Geometry: final body of the model. Coordinates: model frame, mm. Round coordinates to 2 decimals unless told otherwise and drop trailing zeros. Order: outer loops, then holes, each group sorted by start corner. A loop starts at its lowest first (then second) coordinate and runs counter-clockwise, first axis right, second up. Notation, with made-up numbers: (43.5, 67.5) - (66.5, 67.5) arc R18 cw to (66.5, 92.5) - close; hole circle Ø10 at (12.25, 54). An arc over 180 degrees is marked (long way). Put each result on its own line as item: value. Start each with the question number.
(1) Section A-A (z = 25). Output: boundary loops of the cut face in (x, y).
(2) Section B-B (x = -14). Output: boundary loops of the cut face in (y, z).
(3) Pin query (flat end, axial travel): P1, Ø2, axis at x = 46.5, y = 4, coming from the -Z side; P2, Ø2.5, axis at y = 5, z = -2.5, coming from the +X side; P3, Ø1, axis at y = 6, z = -6, coming from the -X side. Return the tip coordinate at first contact, or that it passes through.
(4) Material intervals for L1, parallel to Z at x = 15, y = 4.75; L2, parallel to X at y = 2.75, z = 13, sorted ascending. Write a range as [from, to].
(5) Section C-C (y = 4.75). Output: boundary loops of the cut face in (x, z).
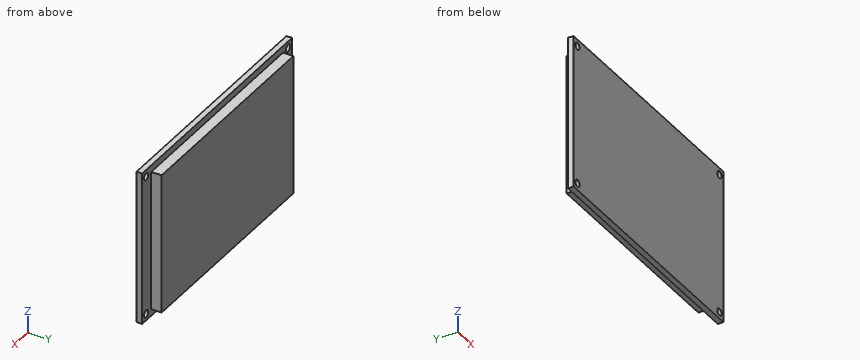
from build123d import *

# Parameters (mm, degrees)
SKETCH1_W                      = 120
SKETCH1_H                      = 74
BOSS_EXTRUDE1_DEPTH            = 2.7
SKETCH2_W                      = 105.56
SKETCH2_H                      = 67.5
BOSS_EXTRUDE2_DEPTH            = 5
M3_CLEARANCE_HOLE1_D           = 3.4
M3_CLEARANCE_HOLE1_CSINK_D     = 3.45
M3_CLEARANCE_HOLE1_CSINK_ANGLE = 90


with BuildPart() as part:
    # Sketch1 → Boss-Extrude1 (new body)
    with BuildSketch(Plane(origin=(0, 0, 0), x_dir=(1, 0, 0), z_dir=(0, 1, 0))):
        Rectangle(SKETCH1_W, SKETCH1_H)
    extrude(amount=BOSS_EXTRUDE1_DEPTH)

    # Sketch2 → Boss-Extrude2 (add)
    with BuildSketch(Plane(origin=(0, 2.7, 0), x_dir=(1, 0, 0), z_dir=(0, 1, 0))):
        Rectangle(SKETCH2_W, SKETCH2_H)
    extrude(amount=BOSS_EXTRUDE2_DEPTH)

    # M3 Clearance Hole1 (through all)
    with Locations(Plane(origin=(0, 2.7, 0), x_dir=(1, 0, 0), z_dir=(0, 1, 0))):
        with Locations((-56.845, 33.735), (56.845, 33.735), (56.845, -33.735), (-56.845, -33.735)):
            CounterSinkHole(M3_CLEARANCE_HOLE1_D / 2, M3_CLEARANCE_HOLE1_CSINK_D / 2, counter_sink_angle=M3_CLEARANCE_HOLE1_CSINK_ANGLE)


solid = part.part
Checks:
1. outline: (-60, 0) - (60, 0) - (60, 2.7) - (52.78, 2.7) - (52.78, 7.7) - (-52.78, 7.7) - (-52.78, 2.7) - (-60, 2.7) - close
2. outline: (0, -37) - (2.7, -37) - (2.7, -33.75) - (7.7, -33.75) - (7.7, 33.75) - (2.7, 33.75) - (2.7, 37) - (0, 37) - close
3. P1: stops at z = -33.75
3. P2: stops at x = 52.78
3. P3: stops at x = -52.78
4. L1: z = [-33.75, 33.75]
4. L2: x = [-52.78, 52.78]
5. outline: (-52.78, -33.75) - (52.78, -33.75) - (52.78, 33.75) - (-52.78, 33.75) - close
